Geometry check sheet. Reference: the model listing, model coordinates, mm. Face numbers are marked on the shaded views. A direction names the side the tool comes from. Coordinates: 2 decimals unless noted, no trailing zeros. Use CSV: the item, a comma, the result in double quotes. Start each with the question number.
1) Depth check by flat-ended pin: P1, Ø3.5, axis at x = -5.15, z = 10.13, coming from the -Y side; P2, Ø6, axis at x = 3.5, z = 28.5, coming from the -Y side; P3, Ø1, axis at x = -2, z = 21, coming from the -Y side. Enter the tip coordinate at first touch or a pass-through.
2) Tool access check on the marked faces 1, 2 and 3. Record the directions out of +Z, -Z, +X, -X, +Y, -Y that give a thin tool (end or side, any length) a straight path to the whole face; none if there is none.
3) Draft check along X on the marked faces 4, 5 and 6. Enter one of: released by +X, released by -X, zero draft, split by the parting line, or undercut.
4) Thickness scan on probe 1 along Y at (x, z) = (0, 1.5) (3 decimals); probe 2 along X at (y, z) = (19.05, 2) (1 decimal); probe 3 along X at (y, z) = (19, 9). Record the ranges inside material, lowest first. Write a range as [from, to].
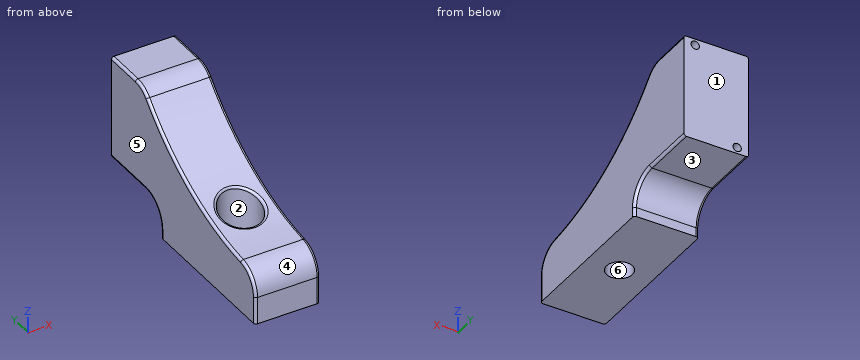
from build123d import *

# Parameters (mm, degrees)
BOSS_EXTRUDE1_DEPTH     = 7.9375
CUT_EXTRUDE1_DEPTH      = 69.000110012
CUT_EXTRUDE1_DEPTH_BACK = 69.000110012
SKETCH2_R               = 3.175
CUT_EXTRUDE4_START      = 6.35
SKETCH2_3_R             = 5.08
SKETCH2_3_R_2           = 3.175
CUT_EXTRUDE4_DEPTH      = 62.650110074
SKETCH3_R               = 1.016
CUT_EXTRUDE2_DEPTH      = 12.7
FILLET1_R               = 6.35
FILLET2_R               = 0.635


with BuildPart() as part:
    # Sketch1 → Boss-Extrude1 (new, symmetric)
    with BuildSketch(Plane(origin=(0, 0, 0), x_dir=(0, 0, -1), z_dir=(1, 0, 0))):
        with BuildLine():
            Line((-12.7, 0), (0, 0))
            Line((0, 0), (0, 38.1))
            Line((0, 38.1), (-8.603985801, 38.1))
            Line((-8.603985801, 38.1), (-8.603985801, 58.35015))
            Line((-8.603985801, 58.35015), (-34.003985801, 58.35015))
            Line((-34.003985801, 58.35015), (-34.003985801, 45.65015))
            ThreePointArc((-34.003985801, 45.65015), (-18.28813969, 25.18827111), (-12.7, 0))
        make_face()
    extrude(amount=BOSS_EXTRUDE1_DEPTH, both=True)

    # Sketch2 → Cut-Extrude1 (cut, two sides: drawn at the far end of the back side and taken through both)
    with BuildSketch(Plane.XY.offset(-CUT_EXTRUDE1_DEPTH_BACK)):
        with Locations((0, 19.05)):
            Circle(SKETCH2_R)
    extrude(amount=CUT_EXTRUDE1_DEPTH + CUT_EXTRUDE1_DEPTH_BACK, mode=Mode.SUBTRACT)

    # Sketch2_3 → Cut-Extrude4 (cut, through all)
    with BuildSketch(Plane.XY.offset(CUT_EXTRUDE4_START)):
        with Locations(Location((0, 19.05, 0), (0, 0, 180))):
            Circle(SKETCH2_3_R)
        with Locations((0, 19.05)):
            Circle(SKETCH2_3_R_2, mode=Mode.SUBTRACT)
    extrude(amount=CUT_EXTRUDE4_DEPTH, mode=Mode.SUBTRACT)

    # Sketch3 → Cut-Extrude2 (cut)
    with BuildSketch(Plane(origin=(0, 58.35015, 0), x_dir=(1, 0, 0), z_dir=(0, 1, 0))):
        with Locations(Location((-5.14985, -10.128440702, 0), (0, 0, 270))):
            Circle(SKETCH3_R)
        with Locations(Location((5.14985, -32.479530901, 0), (0, 0, 270))):
            Circle(SKETCH3_R)
    extrude(amount=-CUT_EXTRUDE2_DEPTH, mode=Mode.SUBTRACT)

    # Fillet1
    fillet1_edges = [part.edges().sort_by_distance(p)[0] for p in [
        (0, 38.1, 8.603985801),
        (0, 0, 12.7),
        (0, 45.65015, 34.003985801),
    ]]
    fillet(fillet1_edges, radius=FILLET1_R)

    # Fillet2
    fillet2_edges = [part.edges().sort_by_distance(p)[0] for p in [
        (7.9375, 51.400075, 8.603985801),
        (5.07889774, 19.155819442, 15.864451693),
        (-7.9375, 0, 3.328298297),
        (7.9375, 0, 3.328298297),
        (-7.9375, 53.436653755, 34.003985801),
        (-7.9375, 38.1, 1.126992901),
        (-7.9375, 26.546479972, 18.943050417),
        (-7.9375, 45.970406475, 33.468275281),
        (-7.9375, 1.648552323, 10.924955733),
        (7.9375, 26.546479972, 18.943050417),
        (7.9375, 53.436653755, 34.003985801),
        (7.9375, 38.1, 1.126992901),
        (7.9375, 45.970406475, 33.468275281),
        (7.9375, 1.648552323, 10.924955733),
        (-7.9375, 39.959871939, 6.744113862),
        (7.9375, 39.959871939, 6.744113862),
        (-7.9375, 51.400075, 8.603985801),
    ]]
    fillet(fillet2_edges, radius=FILLET2_R)


solid = part.part
Evaluation:
1,P1,"y = 0.24"
1,P2,"y = 36.89"
1,P3,"y = 29.47"
2,face 1,"+Z, -Z, +X, -X, +Y"
2,face 2,"+Z"
2,face 3,"-Z, +X, -X, +Y"
3,face 4,"zero draft"
3,face 5,"released by -X"
3,face 6,"undercut"
4,probe 1,"[0, 15.875], [22.225, 38.1]"
4,probe 2,"[-7.9, -3.2], [3.2, 7.9]"
4,probe 3,"[-7.94, -5.08], [5.08, 7.94]"
